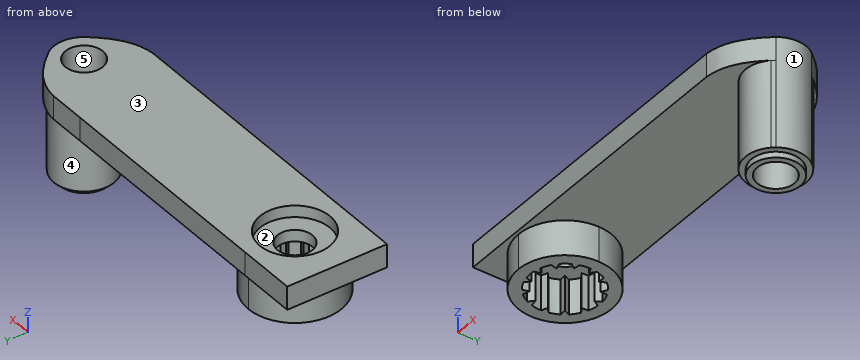
```python
from build123d import *

# Parameters (mm, degrees)
ESBO_O1_R                 = 3
ESBO_O1_R_2               = 1.6
RESSALTO_EXTRUS_O1_DEPTH  = 2
ESBO_O1_4_R               = 3
ESBO_O1_4_R_2             = 1.5
RESSALTO_EXTRUS_O2_DEPTH  = 1
RESSALTO_EXTRUS_O3_START  = -7.5
ESBO_O1_5_R               = 1.6
RESSALTO_EXTRUS_O3_DEPTH  = 7.5
RESSALTO_EXTRUS_O18_START = -3
RESSALTO_EXTRUS_O18_DEPTH = 3
RESSALTO_EXTRUS_O21_START = -8
ESBO_O1_12_R              = 2.1
ESBO_O1_12_R_2            = 1.6
RESSALTO_EXTRUS_O21_DEPTH = 8
RESSALTO_EXTRUS_O22_DEPTH = 3
PADR_OCIRCULAR4_COUNT     = 13


with BuildPart() as part:
    # Esboço1 → Ressalto-extrusão1 (new body)
    with BuildSketch(Plane.XY):
        with BuildLine():
            add(Edge.make_bspline(
                [(3.201918926, -9.498277946), (5.089880376, -9.374786464), (6.418020478, -8.208302927), (7.603254861, -6.751780151)],
                knots=[0.106795249, 0.106795249, 0.106795249, 0.106795249, 1, 1, 1, 1], degree=3))
            ThreePointArc((7.603254861, -6.751780151), (8.1, -5.223277946), (7.603254861, -3.694775741))
            add(Edge.make_bspline(
                [(7.603254861, -3.694775741), (6.423329127, -2.244776711), (5.101774953, -1.082224575), (3.227253733, -0.95)],
                knots=[0.946595223, 0.946595223, 0.946595223, 0.946595223, 1.835799322, 1.835799322, 1.835799322, 1.835799322], degree=3))
            Line((3.227253733, -0.95), (0.099999924, -0.95))
            Line((0.099999924, -0.95), (-19.5, -0.948277946))
            Line((-19.5, -0.948277946), (-24.5, -0.948277946))
            Line((-24.5, -0.948277946), (-24.5, -9.498277946))
            Line((-24.5, -9.498277946), (3.201918926, -9.498277946))
        make_face()
        with Locations((-19.5, -5.223277946)):
            Circle(ESBO_O1_R, mode=Mode.SUBTRACT)
        with Locations((5.5, -5.223277946)):
            Circle(ESBO_O1_R_2, mode=Mode.SUBTRACT)
    extrude(amount=RESSALTO_EXTRUS_O1_DEPTH)

    # Esboço1<4> → Ressalto-extrusão2 (add)
    with BuildSketch(Plane.XY):
        with Locations((-19.5, -5.223277946)):
            Circle(ESBO_O1_4_R)
        with Locations((-19.5, -5.223277946)):
            Circle(ESBO_O1_4_R_2, mode=Mode.SUBTRACT)
    extrude(amount=RESSALTO_EXTRUS_O2_DEPTH)

    # Esboço1<5> → Ressalto-extrusão3 (add)
    with BuildSketch(Plane.XY.offset(RESSALTO_EXTRUS_O3_START)):
        with BuildLine():
            ThreePointArc((7.389037399, -3.436790413), (2.9, -5.223277946), (7.389037399, -7.009765479))
            add(Edge.make_bspline(
                [(7.389037399, -7.009765479), (7.461013495, -6.924914508), (7.532389611, -6.838865753), (7.603254861, -6.751780151)],
                knots=[0.946595223, 0.946595223, 0.946595223, 0.946595223, 1, 1, 1, 1], degree=3))
            ThreePointArc((7.603254861, -6.751780151), (8.1, -5.223277946), (7.603254861, -3.694775741))
            add(Edge.make_bspline(
                [(7.389037399, -3.436790413), (7.461013495, -3.521641384), (7.532389611, -3.607690139), (7.603254861, -3.694775741)],
                knots=[0.946595223, 0.946595223, 0.946595223, 0.946595223, 1, 1, 1, 1], degree=3))
        make_face()
        with Locations((5.5, -5.223277946)):
            Circle(ESBO_O1_5_R, mode=Mode.SUBTRACT)
    extrude(amount=RESSALTO_EXTRUS_O3_DEPTH)

    # Esboço1<10> → Ressalto-extrusão18 (add)
    with BuildSketch(Plane.XY.offset(RESSALTO_EXTRUS_O18_START)):
        with BuildLine():
            ThreePointArc((-19.5, -1.223277946), (-23.5, -5.223277946), (-19.5, -9.223277946))
            Line((-19.5, -9.223277946), (-19.5, -8.223277946))
            ThreePointArc((-19.5, -8.223277946), (-22.5, -5.223277946), (-19.5, -2.223277946))
            Line((-19.5, -2.223277946), (-19.5, -1.223277946))
        make_face()
        with BuildLine():
            Line((-19.5, -8.223277946), (-19.5, -9.223277946))
            ThreePointArc((-19.5, -9.223277946), (-16.671572875, -8.051705071), (-15.5, -5.223277946))
            ThreePointArc((-15.5, -5.223277946), (-16.671572875, -2.394850821), (-19.5, -1.223277946))
            Line((-19.5, -1.223277946), (-19.5, -2.223277946))
            ThreePointArc((-19.5, -2.223277946), (-17.378679656, -3.101957603), (-16.5, -5.223277946))
            ThreePointArc((-16.5, -5.223277946), (-17.378679656, -7.34459829), (-19.5, -8.223277946))
        make_face()
    extrude(amount=RESSALTO_EXTRUS_O18_DEPTH)

    # Esboço1<12> → Ressalto-extrusão21 (add)
    with BuildSketch(Plane.XY.offset(RESSALTO_EXTRUS_O21_START)):
        with Locations((5.5, -5.223277946)):
            Circle(ESBO_O1_12_R)
        with Locations((5.5, -5.223277946)):
            Circle(ESBO_O1_12_R_2, mode=Mode.SUBTRACT)
    extrude(amount=RESSALTO_EXTRUS_O21_DEPTH)

    # Esboço4 → Ressalto-extrusão22 (add)
    with BuildSketch(Plane(origin=(0, 0, -3), x_dir=(-1, 0, 0), z_dir=(0, 0, -1))):
        with BuildLine():
            Line((16.861766136, -3.795089556), (17.42229309, -3.832074862))
            Line((17.42229309, -3.832074862), (17.007212736, -3.554142944))
            ThreePointArc((17.007212736, -3.554142944), (16.931662352, -3.67290969), (16.861766136, -3.795089556))
        make_face()
        with BuildLine():
            Line((17.007212736, -3.554142944), (17.42229309, -3.832074862))
            Line((17.42229309, -3.832074862), (17.422825904, -3.832110019))
            Line((17.422825904, -3.832110019), (17.174502722, -3.328004244))
            ThreePointArc((17.174502722, -3.328004244), (17.088205821, -3.439111799), (17.007212736, -3.554142944))
        make_face()
    ressalto_extrus_o22 = extrude(amount=-RESSALTO_EXTRUS_O22_DEPTH)

    # PadrãoCircular4: Ressalto-extrusão22 ×13 about axis
    padr_ocircular4_axis = Axis((-19.5, -5.223277946, 0), (0, 0, 1))
    for i in range(1, PADR_OCIRCULAR4_COUNT):
        add(ressalto_extrus_o22.rotate(padr_ocircular4_axis, i * 360 / PADR_OCIRCULAR4_COUNT))


solid = part.part
```
Geometry: final body of the model. Coordinates: model frame, mm. Face numbers are marked on the shaded views. A direction names the side the tool comes from. Round coordinates to 2 decimals unless told otherwise and drop trailing zeros. Write each loop counter-clockwise with the first axis right and the second up, starting at its lowest first coordinate (ties: lowest second). Pieces come first, ordered by that corner, then holes.
Item 1: Mould query, pull axis X, two halves, no side actions, for the marked faces 1, 2 and 3. Classes: +X half, -X half, draft (parallel to the pull), parting line (faces both ways), or undercut.
Item 2: Section query A-A (x = -9). Return loops of the section in (y, z), plus the area to 3 significant figures.
Item 3: Material intervals for L1, parallel to Y at x = 5.5, z = -3.5; L2, parallel to X at y = -5.75, z = -2.75; L3, parallel to Y at x = -19.5, z = 0.6, sorted ascending.
Item 4: Pin query (flat end, axial travel): P1, Ø4, axis at x = 5, y = -4.5, coming from the -Z side; P2, Ø5, axis at x = -19.5, y = -5.22, coming from the +Z side; P3, Ø2, axis at x = -10.5, y = -7.5, coming from the -Z side; P4, Ø1, axis at x = -14, z = -3.5, coming from the -Y side. Return the tip coordinate at first contact, or that it passes through.
Item 5: Set-up query: the marked faces 4 and 5. Return all of +Z, -Z, +X, -X, +Y, -Y with unobstructed straight access to the full face (end or side cutting, diameter ignored); none if empty.
Completed:
1. face 1: +X half
1. face 2: undercut
1. face 3: draft
2. outline: (-9.5, 0) - (-0.95, 0) - (-0.95, 2) - (-9.5, 2) - close
2. area: 17.1 mm2
3. L1: y = -7.82 to -6.82, -3.62 to -2.62
3. L2: x = -23.47 to -22.45, -16.55 to -15.53, 2.95 to 3.99, 7.01 to 8.05
3. L3: y = -9.5 to -6.72, -3.72 to -0.95
4. P1: stops at z = -8
4. P2: stops at z = 1
4. P3: stops at z = 0
4. P4: passes through
5. face 4: -Z
5. face 5: +Z, -Z
